Could you check a few things on this model? Use its own coordinates, in mm. Round coordinates to 2 decimals unless told otherwise and drop trailing zeros. Loops run counter-clockwise (first coordinate to the right, second up) from the corner with the lowest first, then second, coordinate; pieces in that order, holes last. Notation, with made-up numbers: (75, 10) - (87, 10) arc R10 cw to (87, 27) - close; hole circle Ø4 at (-29.5, 25.5). An arc over 180 degrees is marked (long way). Use one line per item in the form item = value.
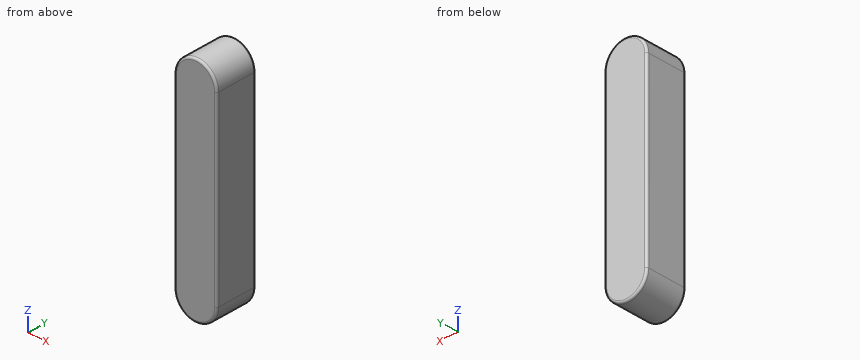
```python
from build123d import *

# Parameters (mm, degrees)
BOSS_EXTRUDE1_START = 2.38125
BOSS_EXTRUDE1_DEPTH = 4.7625
FILLET1_R           = 0.238125


with BuildPart() as part:
    # Sketch4 → Boss-Extrude1 (new body)
    with BuildSketch(Plane(origin=(0, 0, 0), x_dir=(1, 0, 0), z_dir=(0, 1, 0)).offset(BOSS_EXTRUDE1_START)):
        with BuildLine():
            Line((-2.38125, 10.31875), (-2.38125, -10.31875))
            ThreePointArc((-2.38125, -10.31875), (0, -12.7), (2.38125, -10.31875))
            Line((2.38125, -10.31875), (2.38125, 10.31875))
            ThreePointArc((2.38125, 10.31875), (0, 12.7), (-2.38125, 10.31875))
        make_face()
    extrude(amount=-BOSS_EXTRUDE1_DEPTH)

    # Fillet1
    fillet1_edges = [part.edges().sort_by_distance(p)[0] for p in [
        (0, -2.38125, 12.7),
        (2.38125, -2.38125, 0),
        (0, -2.38125, -12.7),
        (2.38125, 2.38125, 0),
        (0, 2.38125, 12.7),
        (-2.38125, 2.38125, 0),
        (0, 2.38125, -12.7),
        (-2.38125, -2.38125, 0),
    ]]
    fillet(fillet1_edges, radius=FILLET1_R)


solid = part.part
```
1. If we section it at A-A, the plane y = 1.4: Write out the boundary of the cut face in (x, z).
Solution:
outline = (-2.38, -10.32) arc R2.38 ccw to (2.38, -10.32) - (2.38, 10.32) arc R2.38 ccw to (-2.38, 10.32) - close
2. For P1, Ø1, axis at x = -1, y = -1.5, coming from the +Z side; P2, Ø1, axis at x = 1.5, y = 1, coming from the +Z side, each with a flat end and sliding along its axis, tell me the tip position at first contact or that it passes through.
Solution:
P1 = 12.65
P2 = 12.48
3. Please list where these lines run through material, in increasing order: line 1 along Z through (x, y) = (0.1, -0.45); line 2 along Z through (x, y) = (1.35, 1.55); line 3 along X through (y, z) = (-2.2, -11).
Solution:
line_1 = -12.7 to 12.7
line_2 = -12.28 to 12.28
line_3 = -2.27 to 2.27
